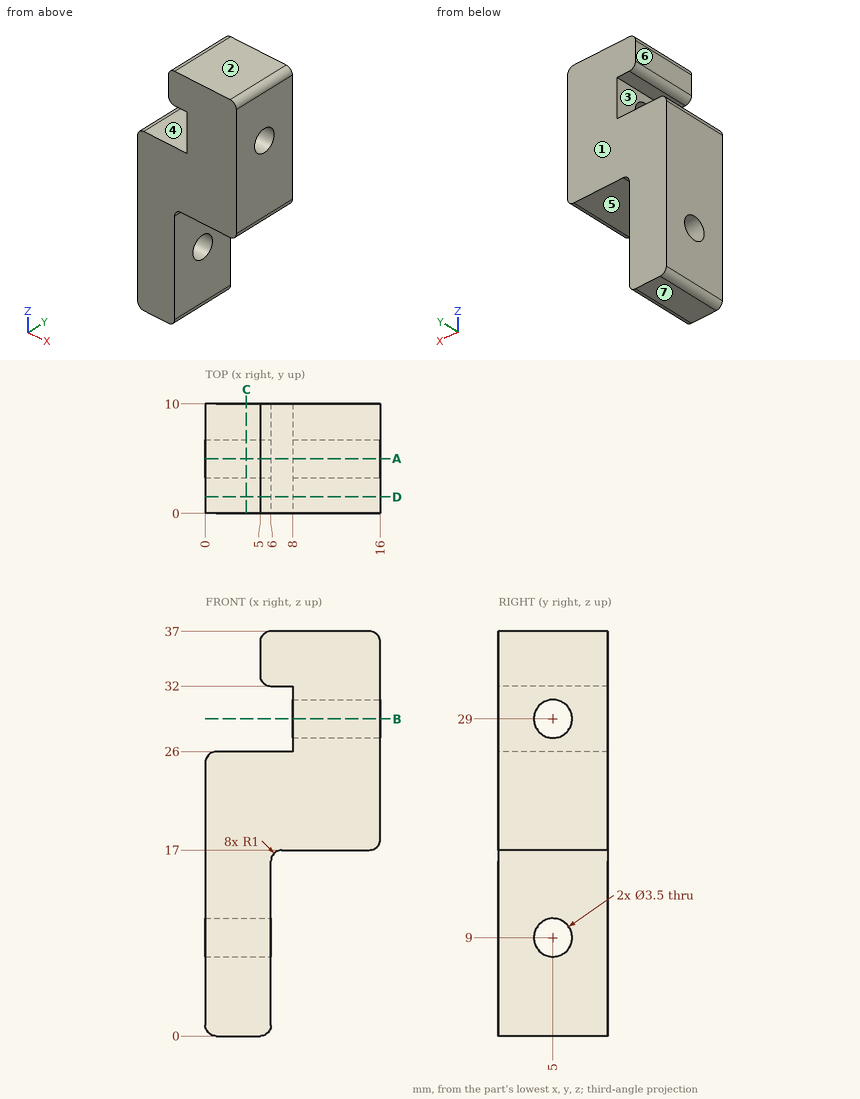
Job drawing, mm, ordinate dimensions from the low corner. One solid piece. A direction names the side the tool comes from. Give positions to 0.01 mm unless a question says otherwise; leave off trailing zeros. Loops run counter-clockwise (first coordinate to the right, second up) from the corner with the lowest first, then second, coordinate; pieces in that order, holes last. Notation, with made-up numbers: (63.25, 49) - (80.25, 49) arc R20 ccw to (80.25, 74) - close; hole circle Ø5 at (42.5, 75.25). An arc over 180 degrees is marked (long way). Use one line per item in the form item = value.
(1) Drop flat-ended pins along their axis: P1, Ø5, axis at y = 3, z = 29, coming from the -X side; P2, Ø4, axis at x = 10.5, y = 3.5, coming from the -Z side; P3, Ø3, axis at y = 3.5, z = 8.5, coming from the +X side. Give the stop position or say it passes through.
Determined:
P1 = 8
P2 = 17
P3 = 6
(2) Pull direction Z, two halves, no side cores. Call the marked faces 1, 2, 3 and 4: pulls with the +Z half, pulls with the -Z half, needs draft (parallel to the pull), parting line crosses it, or undercut.
Determined:
face_1 = needs draft
face_2 = pulls with the +Z half
face_3 = undercut
face_4 = undercut
(3) Cut at B-B (z = 29). Give the cut face in (x, y).
Determined:
outline = (8, 0) - (16, 0) - (16, 3.25) - (8, 3.25) - close; (8, 6.75) - (16, 6.75) - (16, 10) - (8, 10) - close
(4) Cut at A-A (y = 5). Give the cut face in (x, z).
Determined:
outline = (0, 1) arc R1 ccw to (1, 0) - (5, 0) arc R1 ccw to (6, 1) - (6, 7.25) - (0, 7.25) - close; (0, 10.75) - (6, 10.75) - (6, 16) arc R1 cw to (7, 17) - (15, 17) arc R1 ccw to (16, 18) - (16, 27.25) - (8, 27.25) - (8, 26) - (1, 26) arc R1 ccw to (0, 25) - close; (5, 33) arc R1 ccw to (6, 32) - (8, 32) - (8, 30.75) - (16, 30.75) - (16, 36) arc R1 ccw to (15, 37) - (6, 37) arc R1 ccw to (5, 36) - close
(5) Drill centre lines: L1, parallel to Z at x = 10.75, y = 5; L2, parallel to Z at x = 2, y = 5; L3, parallel to Z at x = 1.75, y = 1.75. Where is each one in solid material? Low to high.
Determined:
L1 = 17 to 27.25, 30.75 to 37
L2 = 0 to 7.25, 10.75 to 26
L3 = 0 to 26
(6) Cut at C-C (x = 3.75). Give the cut face in (y, z), then the cut area to 3 significant figures.
Determined:
outline = (0, 0) - (10, 0) - (10, 26) - (0, 26) - close; hole circle Ø3.5 at (5, 9)
area = 250 mm^2
(7) Cut at D-D (y = 1.5). Give the cut face in (x, z).
Determined:
outline = (0, 1) arc R1 ccw to (1, 0) - (5, 0) arc R1 ccw to (6, 1) - (6, 16) arc R1 cw to (7, 17) - (15, 17) arc R1 ccw to (16, 18) - (16, 36) arc R1 ccw to (15, 37) - (6, 37) arc R1 ccw to (5, 36) - (5, 33) arc R1 ccw to (6, 32) - (8, 32) - (8, 26) - (1, 26) arc R1 ccw to (0, 25) - close
(8) 3-axis set-ups, long thin cutter, end or side, ignore diameter. For the marked faces 5, 6 and 7: which of +Z, -Z, +X, -X, +Y, -Y reach the whole face in a straight line?
Determined:
face_5 = -Z, +X, +Y, -Y
face_6 = +Z, -X, +Y, -Y
face_7 = -Z, +X, -X, +Y, -Y
